Here's how the part is built. I have some questions about the finished solid (model axes, mm). A direction names the side the tool comes from. Give positions to 0.01 mm unless a question says otherwise; leave off trailing zeros. Loops run counter-clockwise (first coordinate to the right, second up) from the corner with the lowest first, then second, coordinate; pieces in that order, holes last. Notation, with made-up numbers: M 66,30.5 L 104,30.5 A8 ccw 104,38.5 Z; hole C 15,0 d10. An arc over 180 degrees is marked long. Answer as CSV lines item,"result". Start each with the question number.
Item 1: I want a section at C-C on x = 25. List the corners of the cut face in (y, z) for me.
Item 2: I want a section at A-A on z = -25. List the corners of the cut face in (x, y) for me.
Item 3: If I drill on line 1 along X through (y, z) = (19, -25); line 2 along Z through (x, y) = (125, 11.5); line 3 along Z through (x, y) = (25, 30), over which ranges is the centre line in solid material (lowest first)? Write a range as from..to.
Item 4: For faces 4 (the flat face through (14, 0, -25)), 5 (the cylindrical face through (112.987, 25.572, -167.216)), 6 (the flat face through (14, 50, -25)), which set-ups out of +Z, -Z, +X, -X, +Y, -Y let a thin tool reach every point of the face, with its end or its side?
Item 5: Will these pins go through, and if not, where does the flat tip stop? P1, Ø1, axis at y = 34.5, z = -184.5, coming from the +X side; P2, Ø12, axis at x = 28, y = 79, coming from the +Z side; P3, Ø12, axis at x = 125, z = -25, coming from the -Y side; P4, Ø15, axis at y = 20.5, z = -24.5, coming from the -X side.
Item 6: I want a section at B-B on y = 25. List the corners of the cut face in (x, z) for me, plus the area to 3 significant figures.
Item 7: If we mould it in two halves opening along X, with no side actions, what happens to faces 1 (the flat face through (25, 25, 0)), 2 (the cylindrical face through (125.394, 5.528, -105.916)), 3 (the cylindrical face through (117.63, 25.35, -31.76))? For each: released by +X, released by -X, zero draft, split by the parting line, or undercut.
Item 8: I want a section at D-D on x = 129. List the corners of the cut face in (y, z) for me, plus the area to 3 significant figures.
from build123d import *

# Parameters (mm, degrees)
BOSS_EXTRUDE1_DEPTH = 50
SKETCH3_R           = 10
CUT_EXTRUDE1_DEPTH  = 50
SKETCH4_W           = 150
SKETCH4_H           = 50
BOSS_EXTRUDE2_DEPTH = 50
SKETCH5_W           = 150
SKETCH5_H           = 50
BOSS_EXTRUDE3_DEPTH = 50
SKETCH6_W           = 200
SKETCH6_H           = 200
SKETCH6_W_2         = 150
SKETCH6_H_2         = 150
BOSS_EXTRUDE4_DEPTH = 50
SKETCH7_R           = 32
BOSS_EXTRUDE5_DEPTH = 12
SKETCH8_R           = 13
BOSS_EXTRUDE6_DEPTH = 112


with BuildPart() as part:
    # Sketch2 → Boss-Extrude1 (new body)
    with BuildSketch(Plane(origin=(0, 0, 0), x_dir=(1, 0, 0), z_dir=(0, 1, 0))):
        Polygon((0, 100), (0, 0), (50, 0), (50, 50), (100, 50), (100, 0), (150, 0), (150, 100), align=None)
    extrude(amount=BOSS_EXTRUDE1_DEPTH)

    # Sketch3 → Cut-Extrude1 (cut)
    with BuildSketch(Plane(origin=(0, 50, 0), x_dir=(1, 0, 0), z_dir=(0, 1, 0))):
        with Locations((125, 25)):
            Circle(SKETCH3_R)
        with Locations((25, 25)):
            Circle(SKETCH3_R)
    extrude(amount=-CUT_EXTRUDE1_DEPTH, mode=Mode.SUBTRACT)

    # Sketch4 → Boss-Extrude2 (add)
    with BuildSketch(Plane(origin=(0, 50, 0), x_dir=(1, 0, 0), z_dir=(0, 1, 0))):
        with Locations((75, 75)):
            Rectangle(SKETCH4_W, SKETCH4_H)
    extrude(amount=BOSS_EXTRUDE2_DEPTH)

    # Sketch5 → Boss-Extrude3 (add)
    with BuildSketch(Plane.XZ):
        with Locations((75, -75)):
            Rectangle(SKETCH5_W, SKETCH5_H)
    extrude(amount=BOSS_EXTRUDE3_DEPTH)

    # Sketch6 → Boss-Extrude4 (add)
    with BuildSketch(Plane(origin=(0, 0, -100), x_dir=(-1, 0, 0), z_dir=(0, 0, -1))):
        with Locations((-75, 25)):
            Rectangle(SKETCH6_W, SKETCH6_H)
        with Locations((-75, 25)):
            Rectangle(SKETCH6_W_2, SKETCH6_H_2, mode=Mode.SUBTRACT)
    extrude(amount=-BOSS_EXTRUDE4_DEPTH)

    # Sketch7 → Boss-Extrude5 (add)
    with BuildSketch(Plane(origin=(0, 0, -100), x_dir=(-1, 0, 0), z_dir=(0, 0, -1))):
        with Locations((-100, 25)):
            Circle(SKETCH7_R)
    extrude(amount=BOSS_EXTRUDE5_DEPTH)

    # Sketch8 → Boss-Extrude6 (add)
    with BuildSketch(Plane(origin=(0, 0, -112), x_dir=(-1, 0, 0), z_dir=(0, 0, -1))):
        with Locations((-100, 25)):
            Circle(SKETCH8_R)
    extrude(amount=BOSS_EXTRUDE6_DEPTH)


solid = part.part
Result:
1,outline,"M -75,-100 L 125,-100 L 125,-50 L 50,-50 L 50,-35 L 0,-35 L 0,-50 L -75,-50 Z; M 0,-15 L 50,-15 L 50,0 L 0,0 Z"
2,outline,"M 0,0 L 15,0 L 15,50 L 0,50 Z; M 35,0 L 50,0 L 50,50 L 35,50 Z; M 100,0 L 115,0 L 115,50 L 100,50 Z; M 135,0 L 150,0 L 150,50 L 135,50 Z"
3,line 1,"0..15, 35..50, 100..115, 135..150"
3,line 2,"-112..-35, -15..0"
3,line 3,"-100..-35, -15..0"
4,face 4,"+Z, +X, -X, -Y"
4,face 5,"-Z"
4,face 6,"+Z, +X, -X, +Y"
5,P1,"x = 109.38"
5,P2,"z = -50"
5,P3,"through"
5,P4,"x = 0"
6,outline,"M -25,-100 L 68,-100 L 68,-112 L 87,-112 L 87,-224 L 113,-224 L 113,-112 L 132,-112 L 132,-100 L 175,-100 L 175,-50 L 150,-50 L 150,0 L 100,0 L 100,-50 L 50,-50 L 50,0 L 0,0 L 0,-50 L -25,-50 Z; hole C 25,-25 d20; hole C 125,-25 d20"
6,area,"18,100 mm^2"
7,face 1,"zero draft"
7,face 2,"split by the parting line"
7,face 3,"undercut"
8,outline,"M -75,-100 L 11.47,-100 L 11.47,-112 L 38.53,-112 L 38.53,-100 L 125,-100 L 125,-50 L 50,-50 L 50,-34.17 L 0,-34.17 L 0,-50 L -75,-50 Z; M 0,-15.83 L 50,-15.83 L 50,0 L 0,0 Z"
8,area,"11,900 mm^2"
